For this review, take the finished solid that the model builds, in its own axes (mm). Round coordinates to 2 decimals unless told otherwise and drop trailing zeros. Loops run counter-clockwise (first coordinate to the right, second up) from the corner with the lowest first, then second, coordinate; pieces in that order, holes last.
Autodesk Inventor part; units mm, degrees
ref_plane "YZ Plane" through (0, 0, 0) normal (1, 0, 0) x (0, 1, 0)
ref_plane "XZ Plane" through (0, 0, 0) normal (0, 1, 0) x (-1, 0, 0)
ref_plane "XY Plane" through (0, 0, 0) normal (0, 0, 1) x (1, 0, 0)
sketch "Sketch1" plane through (0, 0, 0) normal (0, 0, 1) x (1, 0, 0)
  line L0 (9.1023, -3.4337) -> (9.1023, 0.9663)
  line L1 (6.7023, -3.4337) -> (9.1023, -3.4337)
  line L2 (6.7023, 0.9663) -> (6.7023, -3.4337)
  line L3 (9.1023, 0.9663) -> (6.7023, 0.9663)
  line L4 (-3.672, 5.3) -> (-3.672, 9.4)
  line L5 (17.5929, 9.4) -> (17.5929, -15.6)
  line L6 (17.5929, -15.6) -> (-3.672, -15.6)
  line L7 (-3.672, -15.6) -> (-3.672, 9.4)
  line L8 (-3.672, 9.4) -> (17.5929, 9.4)
  line L9 (17.5929, 9.4) -> (17.5929, -15.6)
  point P0 (0, 0)
extrude "Extrusion1" add sketch "Sketch1" along normal blind 0.7
sketch "Sketch2" plane through (0, 0, 0) normal (0, 0, -1) x (-1, 0, 0)
  line L0 (-17.5929, -15.6) -> (-17.5929, 9.4)
  line L1 (3.672, -15.6) -> (-17.5929, -15.6)
  line L2 (3.672, 9.4) -> (3.672, -15.6)
  line L3 (-17.5929, 9.4) -> (3.672, 9.4)
  line L4 (-9.1023, -3.4337) -> (-6.7023, -3.4337)
  line L5 (-9.1023, 0.9663) -> (-9.1023, -3.4337)
  line L6 (-6.7023, 0.9663) -> (-9.1023, 0.9663)
  line L7 (-6.7023, -3.4337) -> (-6.7023, 0.9663)
  point P0 (0, 0)
extrude "Extrusion2" cut sketch "Sketch2" against normal blind 0.2
sketch "Sketch3" plane through (0, 0, 0.7) normal (0, 0, 1) x (1, 0, 0)
  line L0 (15.9929, 9.4) -> (15.9929, -15.6)
  line L1 (15.9929, -15.6) -> (17.5929, -15.6)
  line L2 (17.5929, 9.4) -> (17.5929, -15.6)
  line L3 (15.9929, 9.4) -> (17.5929, 9.4)
  point P0 (0, 0)
extrude "Extrusion3" cut sketch "Sketch3" against normal through all
properties part number "przod"
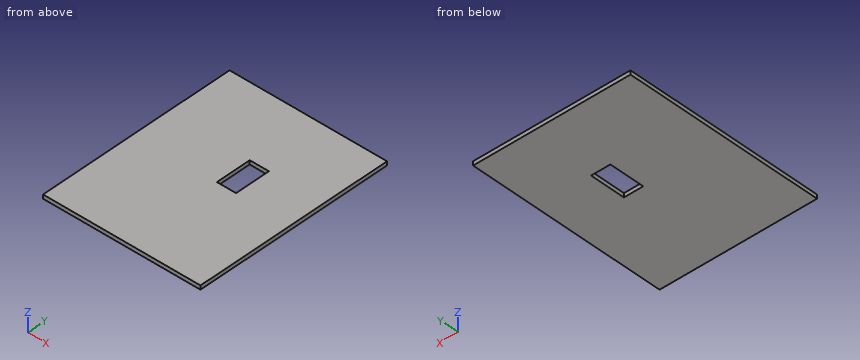
(1) Add section B-B (z = 0.3). Give the boundary of the cut face in (x, y), plus the area to 3 significant figures.
(2) For L1, parallel to Y at x = 8.25, z = 0.5; L2, parallel to X at y = 0.5, z = 0.4, list the stretches that pass through material, from the lowest coordinate up.
(3) Add section A-A (y = -1.25). Give the boundary of the cut face in (x, z).
Outcome:
1. outline: (-3.67, -15.6) - (15.99, -15.6) - (15.99, 9.4) - (-3.67, 9.4) - close; hole (6.7, -3.43) - (9.1, -3.43) - (9.1, 0.97) - (6.7, 0.97) - close
1. area: 481 mm2
2. L1: y = -15.6 to -3.43, 0.97 to 9.4
2. L2: x = -3.67 to 6.7, 9.1 to 15.99
3. outline: (-3.67, 0.2) - (6.7, 0.2) - (6.7, 0.7) - (-3.67, 0.7) - close; (9.1, 0.2) - (15.99, 0.2) - (15.99, 0.7) - (9.1, 0.7) - close
